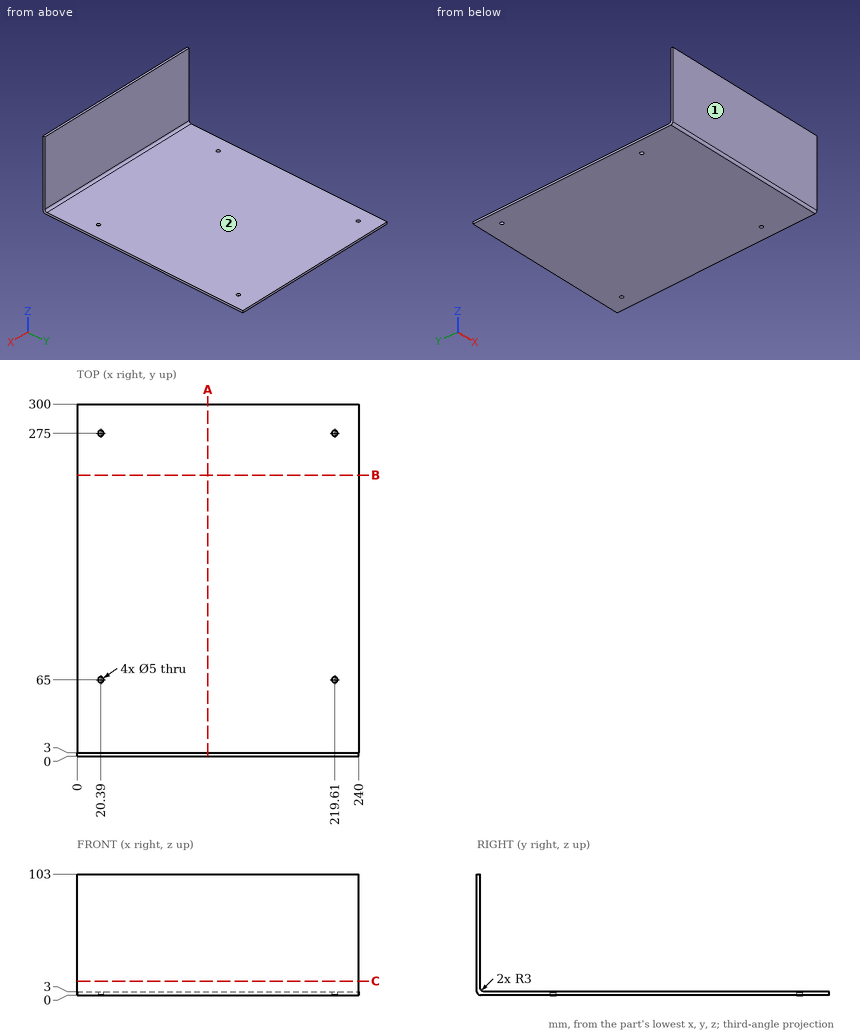
Part print with two shaded views. Sizes in mm from the minimum x, y, z corner. A direction names the side the tool comes from. Round coordinates to 2 decimals unless told otherwise and drop trailing zeros. Write each loop counter-clockwise with the first axis right and the second up, starting at its lowest first coordinate (ties: lowest second). Pieces come first, ordered by that corner, then holes. Notation, with made-up numbers: M -29,38 L -7,38 A12 cw -7,57 Z; hole C 23.25,-31.5 d6. An arc over 180 degrees is marked long. Answer as CSV lines item,"result". Start each with the question number.
1) Band-saw the part on B-B (y = 239.5). List the corners of the cut face in (x, z).
2) Which spindle directions (+Z, -Z, +X, -X, +Y, -Y) get a long thin tool onto all of the face, cutting with end or side? Do the marked faces 1 and 2. Say none if no direction does.
3) Drop a flat-ended pin along its axis: pin 1 (10 mm diameter, centred on x = 67, y = 240, fed in from +Z). Give the stop position or say it passes through.
4) Band-saw the part on A-A (x = 111.5). List the corners of the cut face in (y, z), then the cut area to 3 significant figures.
5) Drill centre lines: L1, parallel to X at y = 65, z = 2; L2, parallel to Y at x = 219.61, z = 1.1; L3, parallel to Y at x = 219.61, z = 2.1. Where is each one in solid material? Low to high.
Worked out:
1,outline,"M 0,0 L 240,0 L 240,3 L 0,3 Z"
2,face 1,"+Z, -Z, +X, -X, -Y"
2,face 2,"+Z, +X, -X, +Y"
3,pin 1,"z = 3"
4,outline,"M 0,3 A3 ccw 3,0 L 300,0 L 300,3 L 6,3 A3 cw 3,6 L 3,103 L 0,103 Z"
4,area,"1,200 mm²"
5,L1,"0 to 17.89, 22.89 to 217.11, 222.11 to 240"
5,L2,"0.68 to 62.5, 67.5 to 272.5, 277.5 to 300"
5,L3,"0.14 to 62.5, 67.5 to 272.5, 277.5 to 300"
